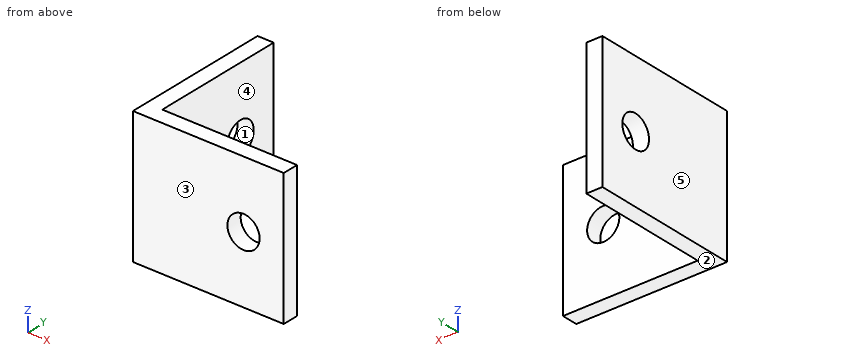
from build123d import *

# Parameters (mm, degrees)
BOSS_EXTRU_1_DEPTH      = 12.7
ESQUISSE2_R             = 1.525
ENL_V_MAT_EXTRU_1_DEPTH = 12.7
ESQUISSE3_R             = 1.525
ENL_V_MAT_EXTRU_2_DEPTH = 12.7


with BuildPart() as part:
    # Esquisse1 → Boss.-Extru.1 (new body)
    with BuildSketch(Plane.XY):
        Polygon((0, 0), (14.27, 0), (14.27, 1.52), (1.52, 1.52), (1.52, 14.27), (0, 14.27), align=None)
    extrude(amount=BOSS_EXTRU_1_DEPTH)

    # Esquisse2 → Enlèv. mat.-Extru.1 (cut)
    with BuildSketch(Plane(origin=(1.52, 0, 0), x_dir=(0, 0, -1), z_dir=(1, 0, 0))):
        with Locations(Location((-6.35, 10.46, 0), (0, 0, 90))):
            Circle(ESQUISSE2_R)
    extrude(amount=-ENL_V_MAT_EXTRU_1_DEPTH, mode=Mode.SUBTRACT)

    # Esquisse3 → Enlèv. mat.-Extru.2 (cut)
    with BuildSketch(Plane(origin=(0, 1.52, 0), x_dir=(1, 0, 0), z_dir=(0, 1, 0))):
        with Locations(Location((10.46, -6.35, 0), (0, 0, 180))):
            Circle(ESQUISSE3_R)
    extrude(amount=-ENL_V_MAT_EXTRU_2_DEPTH, mode=Mode.SUBTRACT)


solid = part.part
Verification items for the finished model (mm, model axes). Face numbers are marked on the shaded views. A direction names the side the tool comes from. Give positions to 0.01 mm unless a question says otherwise; leave off trailing zeros. Write each loop counter-clockwise with the first axis right and the second up, starting at its lowest first coordinate (ties: lowest second). Pieces come first, ordered by that corner, then holes. Notation, with made-up numbers: M -19,-20 L -4,-20 A27 ccw -4,19 Z; hole C 18,67.25 d3. An arc over 180 degrees is marked long. Put each result on its own line as item: value. Start each with the question number.
1. Section check A-A (y = 10.46). Record the cut outline in (x, z) (3 decimals).
2. Section check D-D (z = 3.25). Record the cut outline in (x, y), and give its area (3 significant figures).
3. Scan lines: line 1 along Z through (x, y) = (10.46, 1.1) (3 decimals); line 2 along X through (y, z) = (4.25, 6.75). Record each from-to range of solid material in increasing order. Write a range as [from, to].
4. Section check C-C (z = 6.35). Record the cut outline in (x, y) (3 decimals), and give its area (3 significant figures).
5. Go/stop test with a flat-tipped pin: pin 1 Ø6.5 at (y, z) = (6.5, 9) entering from +X. Record where the tip stops, or that it passes through.
6. Draft check along Y on the marked faces 1, 2 and 3. Enter one of: +Y half, -Y half, draft (parallel to the pull), parting line (faces both ways), or undercut.
7. Set-up check for the marked faces 4 and 5: record each of +Z, -Z, +X, -X, +Y, -Y from which the full face is reachable in a straight line by a thin tool's end or side.
Answer list:
1. outline: M 0,0 L 1.52,0 L 1.52,4.825 L 0,4.825 Z; M 0,7.875 L 1.52,7.875 L 1.52,12.7 L 0,12.7 Z
2. outline: M 0,0 L 14.27,0 L 14.27,1.52 L 1.52,1.52 L 1.52,14.27 L 0,14.27 Z
2. area: 41.1 mm2
3. line 1: [0, 4.825], [7.875, 12.7]
3. line 2: [0, 1.52]
4. outline: M 0,0 L 8.935,0 L 8.935,1.52 L 1.52,1.52 L 1.52,8.935 L 0,8.935 Z; M 0,11.985 L 1.52,11.985 L 1.52,14.27 L 0,14.27 Z; M 11.985,0 L 14.27,0 L 14.27,1.52 L 11.985,1.52 Z
4. area: 31.8 mm2
5. pin 1: x = 1.52
6. face 1: undercut
6. face 2: draft
6. face 3: -Y half
7. face 4: +Z, -Z, +X, +Y
7. face 5: +Z, -Z, -X, +Y, -Y
